```python
from build123d import *

# Parameters (mm, degrees)
SKETCH1_W           = 102
SKETCH1_H           = 10.8
BOSS_EXTRUDE1_DEPTH = 1.2
SKETCH2_W           = 10.8
SKETCH2_H           = 102
BOSS_EXTRUDE2_DEPTH = 160


with BuildPart() as part:
    # Sketch1 → Boss-Extrude1 (new body)
    with BuildSketch(Plane(origin=(0, 0, 0), x_dir=(0, 1, 0), z_dir=(0, 0, 1))):
        with Locations((51, 5.4)):
            Rectangle(SKETCH1_W, SKETCH1_H)
    extrude(amount=BOSS_EXTRUDE1_DEPTH)

    # Sketch2 → Boss-Extrude2 (add)
    with BuildSketch(Plane.XY.offset(1.2)):
        with Locations((-5.4, 51)):
            Rectangle(SKETCH2_W, SKETCH2_H)
        Polygon((-9.2, 100), (-8.4, 100), (-8.4, 96), (-7.4, 96), (-7.4, 100), (-3.4, 100), (-3.4, 96), (-2.4, 96), (-2.4, 100), (-1.6, 100), (-1.6, 2), (-2.4, 2), (-2.4, 6), (-3.4, 6), (-3.4, 2), (-7.4, 2), (-7.4, 6), (-8.4, 6), (-8.4, 2), (-9.2, 2), align=None, mode=Mode.SUBTRACT)
    extrude(amount=BOSS_EXTRUDE2_DEPTH)


solid = part.part
```
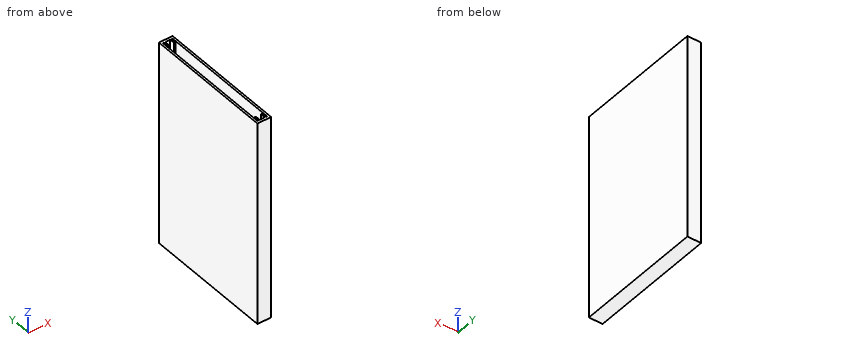
Geometry check sheet. Reference: the model listing, model coordinates, mm. Give positions to 0.01 mm unless a question says otherwise; leave off trailing zeros. Loops run counter-clockwise (first coordinate to the right, second up) from the corner with the lowest first, then second, coordinate; pieces in that order, holes last. Notation, with made-up numbers: (67.5, 13.5) - (84.5, 13.5) arc R32 cw to (84.5, 40.5) - close; hole circle Ø8 at (5, -19.5). An arc over 180 degrees is marked (long way). Use CSV: the item, a comma, the result in double quotes. Start each with the question number.
Q1. Section check B-B, the plane x = -5.75. Record the cut outline in (y, z), and give its area (3 significant figures).
Q2. Go/stop test with a flat-tipped pin: pin 1 Ø1.5 at (y, z) = (36, 101.5) entering from +X. Record where the tip stops, or that it passes through.
Q3. Scan lines: probe 1 along X at (y, z) = (96.5, 10); probe 2 along Y at (x, z) = (-3.5, 47); probe 3 along X at (y, z) = (65, 91.5). Record each from-to range of solid material in increasing order. Write a range as from..to.
Q4. Section check A-A, the plane z = 16.5. Record the cut outline in (x, y).
Q5. Section check C-C, the plane y = 27.5. Record the cut outline in (x, z).
Findings below:
1,outline,"(0, 0) - (102, 0) - (102, 161.2) - (100, 161.2) - (100, 1.2) - (2, 1.2) - (2, 161.2) - (0, 161.2) - close"
1,area,"762 mm^2"
2,pin 1,"stops at x = 0"
3,probe 1,"x = -10.8..-9.2, -8.4..-7.4, -3.4..-2.4, -1.6..0"
3,probe 2,"y = 0..2, 100..102"
3,probe 3,"x = -10.8..-9.2, -1.6..0"
4,outline,"(-10.8, 0) - (0, 0) - (0, 102) - (-10.8, 102) - close; hole (-9.2, 2) - (-8.4, 2) - (-8.4, 6) - (-7.4, 6) - (-7.4, 2) - (-3.4, 2) - (-3.4, 6) - (-2.4, 6) - (-2.4, 2) - (-1.6, 2) - (-1.6, 100) - (-2.4, 100) - (-2.4, 96) - (-3.4, 96) - (-3.4, 100) - (-7.4, 100) - (-7.4, 96) - (-8.4, 96) - (-8.4, 100) - (-9.2, 100) - close"
5,outline,"(-10.8, 0) - (0, 0) - (0, 161.2) - (-1.6, 161.2) - (-1.6, 1.2) - (-9.2, 1.2) - (-9.2, 161.2) - (-10.8, 161.2) - close"
